The model under review builds one solid part; all positions refer to its coordinate system, in mm. Face numbers are marked on the shaded views. A direction names the side the tool comes from. Give positions to 0.01 mm unless a question says otherwise; leave off trailing zeros. Write each loop counter-clockwise with the first axis right and the second up, starting at its lowest first coordinate (ties: lowest second). Pieces come first, ordered by that corner, then holes.
from build123d import *

# Parameters (mm, degrees)
SKETCH_W   = 40
SKETCH_H   = 40
SKETCH_W_2 = 34
SKETCH_H_2 = 34
PAD_DEPTH  = 100
FILLET_R   = 1


with BuildPart() as part:
    # Sketch → Pad (new body)
    with BuildSketch(Plane.XY):
        Rectangle(SKETCH_W, SKETCH_H)
        Rectangle(SKETCH_W_2, SKETCH_H_2, mode=Mode.SUBTRACT)
    extrude(amount=PAD_DEPTH)

    # Fillet
    fillet_edges = [part.edges().sort_by_distance(p)[0] for p in [
        (20, -20, 50),
        (20, 20, 50),
        (-20, -20, 50),
        (-20, 20, 50),
    ]]
    fillet(fillet_edges, radius=FILLET_R)


solid = part.part
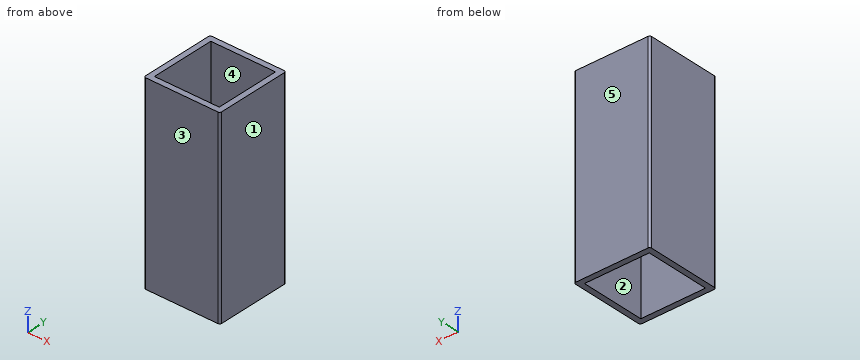
1) Tool access review of the marked faces 4 and 5: name each direction out of +Z, -Z, +X, -X, +Y, -Y from which nothing blocks a thin tool from reaching the whole face with its end or side.
2) Consider section C-C, the plane z = 41. Give the boundary of the cut face in (x, y).
3) Insertion check: pin 1 (5 mm diameter, centred on x = 12, y = -13, fed in from -Z) (3 decimals). The pin has a flat end and moves straight along its axis. Give the tip position at first contact, or say it passes through.
4) The part is to be moulded in two halves that separate along Y. For the marked faces 1, 2 and 3, say which applies: +Y half, -Y half, draft (parallel to the pull), parting line (faces both ways), or undercut.
5) Consider section A-A, the plane x = -11. Give the boundary of the cut face in (y, z).
6) To check wall thickness, follow probe 1 along X at (y, z) = (0.5, 18.5). State the ranges of the line that lie inside material, in increasing order.
Answer block:
1. face 4: +Z, -Z
1. face 5: +Z, -Z, +X, -X, +Y
2. outline: (-20, -19) arc R1 ccw to (-19, -20) - (19, -20) arc R1 ccw to (20, -19) - (20, 19) arc R1 ccw to (19, 20) - (-19, 20) arc R1 ccw to (-20, 19) - close; hole (-17, -17) - (17, -17) - (17, 17) - (-17, 17) - close
3. pin 1: passes through
4. face 1: draft
4. face 2: undercut
4. face 3: -Y half
5. outline: (-20, 0) - (-17, 0) - (-17, 100) - (-20, 100) - close; (17, 0) - (20, 0) - (20, 100) - (17, 100) - close
6. probe 1: x = -20 to -17, 17 to 20
